Geometry check sheet. Reference: the model listing, model coordinates, mm. Give positions to 0.01 mm unless a question says otherwise; leave off trailing zeros. Order: outer loops, then holes, each group sorted by start corner. A loop starts at its lowest first (then second) coordinate and runs counter-clockwise, first axis right, second up. Notation, with made-up numbers: M -25.75,23 L 1.25,23 A22 cw 1.25,33 Z; hole C 57,6.25 d7. An arc over 180 degrees is marked long. One line per question, with ' | ' between items. Start each with the question number.
from build123d import *

# Parameters (mm, degrees)
CROQUIS1_R                   = 2.5
SALIENTE_EXTRUIR1_DEPTH      = 4
CROQUIS2_W                   = 50
CROQUIS2_H                   = 4
SALIENTE_EXTRUIR2_DEPTH      = 20
SALIENTE_EXTRUIR3_DEPTH      = 3
SALIENTE_EXTRUIR3_DEPTH_BACK = 53
CROQUIS4_W                   = 23
CROQUIS4_H                   = 20
CORTAR_EXTRUIR1_DEPTH        = 20
CROQUIS5_R                   = 3
CORTAR_EXTRUIR2_DEPTH        = 17
CROQUIS6_R                   = 2.5
CORTAR_EXTRUIR3_DEPTH        = 20


with BuildPart() as part:
    # Croquis1 → Saliente-Extruir1 (new body)
    with BuildSketch(Plane(origin=(0, 0, 0), x_dir=(1, 0, 0), z_dir=(0, 1, 0))):
        Polygon((0, 0), (0, 20), (50, 20), (50, 0), (50, -4), (0, -4), align=None)
        with Locations(Location((10, 10, 0), (0, 0, 270))):
            Circle(CROQUIS1_R, mode=Mode.SUBTRACT)
        with Locations(Location((40, 10, 0), (0, 0, 270))):
            Circle(CROQUIS1_R, mode=Mode.SUBTRACT)
    extrude(amount=SALIENTE_EXTRUIR1_DEPTH)

    # Croquis2 → Saliente-Extruir2 (add)
    with BuildSketch(Plane(origin=(0, 4, 0), x_dir=(1, 0, 0), z_dir=(0, 1, 0))):
        with Locations((25, -2)):
            Rectangle(CROQUIS2_W, CROQUIS2_H)
    extrude(amount=SALIENTE_EXTRUIR2_DEPTH)

    # Croquis3 → Saliente-Extruir3 (add, two sides: drawn at the far end of the back side and taken through both)
    with BuildSketch(Plane.ZY.offset(-SALIENTE_EXTRUIR3_DEPTH_BACK)):
        Polygon((-20, 4), (-20, 0), (4, 0), (4, 24), (0, 24), align=None)
    extrude(amount=SALIENTE_EXTRUIR3_DEPTH + SALIENTE_EXTRUIR3_DEPTH_BACK)

    # Croquis4 → Cortar-Extruir1 (cut)
    with BuildSketch(Plane(origin=(0, 0, -20), x_dir=(-1, 0, 0), z_dir=(0, 0, -1))):
        with Locations((-39, 14)):
            Rectangle(CROQUIS4_W, CROQUIS4_H)
        with Locations((-11, 14)):
            Rectangle(CROQUIS4_W, CROQUIS4_H)
    extrude(amount=-CORTAR_EXTRUIR1_DEPTH, mode=Mode.SUBTRACT)

    # Croquis5 → Cortar-Extruir2 (cut)
    with BuildSketch(Plane(origin=(0, 0, 0), x_dir=(-1, 0, 0), z_dir=(0, 0, -1))):
        with Locations((-40, 14)):
            Circle(CROQUIS5_R)
        with Locations((-10, 14)):
            Circle(CROQUIS5_R)
    extrude(amount=-CORTAR_EXTRUIR2_DEPTH, mode=Mode.SUBTRACT)

    # Croquis6 → Cortar-Extruir3 (cut)
    with BuildSketch(Plane(origin=(0, 4, 0), x_dir=(1, 0, 0), z_dir=(0, 1, 0))):
        with Locations(Location((10, 10, 0), (0, 0, 180))):
            Circle(CROQUIS6_R)
        with Locations(Location((40, 10, 0), (0, 0, 180))):
            Circle(CROQUIS6_R)
    extrude(amount=-CORTAR_EXTRUIR3_DEPTH, mode=Mode.SUBTRACT)

    # Croquis7 → Cortar-Revolución1 (revolve, cut)
    with BuildSketch(Plane.XY.offset(-10), mode=Mode.PRIVATE) as cortar_revoluci_n1_sk:
        Polygon((40, 0.7), (37.5, 0.7), (34.2, 4), (40, 4), align=None)
    revolve(cortar_revoluci_n1_sk.sketch.rotate(Axis((40, 0.7, -10), (0, 1, 0)), 270), axis=Axis((40, 0.7, -10), (0, 1, 0)), mode=Mode.SUBTRACT)

    # Croquis8 → Cortar-Revolución2 (revolve, cut)
    with BuildSketch(Plane.XY.offset(-10), mode=Mode.PRIVATE) as cortar_revoluci_n2_sk:
        Polygon((10, 4), (10, 0.7), (12.5, 0.7), (15.8, 4), align=None)
    revolve(cortar_revoluci_n2_sk.sketch.rotate(Axis((10, 4, -10), (0, -1, 0)), 90), axis=Axis((10, 4, -10), (0, -1, 0)), mode=Mode.SUBTRACT)

    # Croquis9 → Cortar-Revolución3 (revolve, cut)
    with BuildSketch(Plane(origin=(0, 14, 0), x_dir=(1, 0, 0), z_dir=(0, 1, 0)), mode=Mode.PRIVATE) as cortar_revoluci_n3_sk:
        Polygon((40, 0), (40, -3.3), (43, -3.3), (46.3, 0), align=None)
    revolve(cortar_revoluci_n3_sk.sketch.rotate(Axis((40, 14, 0), (0, 0, 1)), 180), axis=Axis((40, 14, 0), (0, 0, 1)), mode=Mode.SUBTRACT)

    # Croquis10 → Cortar-Revolución4 (revolve, cut)
    with BuildSketch(Plane(origin=(0, 14, 0), x_dir=(1, 0, 0), z_dir=(0, 1, 0)), mode=Mode.PRIVATE) as cortar_revoluci_n4_sk:
        Polygon((10, 0), (10, -3.3), (13, -3.3), (16.3, 0), align=None)
    revolve(cortar_revoluci_n4_sk.sketch.rotate(Axis((10, 14, 0), (0, 0, 1)), 180), axis=Axis((10, 14, 0), (0, 0, 1)), mode=Mode.SUBTRACT)


solid = part.part
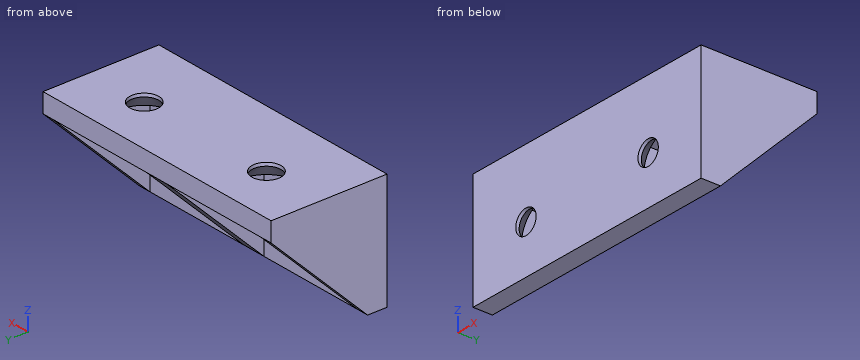
Item 1: Cross-section at C-C, the plane y = 14. Record the cut outline in (x, z).
Item 2: Cross-section at B-B, the plane z = -10. Record the cut outline in (x, y), plus the area to 3 significant figures.
Item 3: Depth check by flat-ended pin: pin 1 (3 mm diameter, centred on x = 47, z = -12, fed in from +Y); pin 2 (6 mm diameter, centred on x = 38.5, y = 18, fed in from -Z); pin 3 (6 mm diameter, centred on x = 11.5, z = -8, fed in from +Y); pin 4 (6 mm diameter, centred on y = 14, z = -17, fed in from -X). Enter the tip coordinate at first touch or a pass-through.
Item 4: Cross-section at D-D, the plane z = -3. Record the cut outline in (x, y), plus the area to 3 significant figures.
Item 5: Material ranges on line 1 along X through (y, z) = (0.2, -10); line 2 along X through (y, z) = (17.25, -6); line 3 along Y through (x, z) = (40, 3.8), recorded low to high.
Item 6: Cross-section at A-A, the plane x = 40. Record the cut outline in (y, z).
Outcome:
1) outline: M -3,-10 L -0.5,-10 L -0.5,0 L 3.7,0 L 7,3.3 L 7,4 L -3,4 Z; M 13,3.3 L 16.3,0 L 22.5,0 L 22.5,-10 L 27.5,-10 L 27.5,0 L 33.7,0 L 37,3.3 L 37,4 L 13,4 Z; M 43,3.3 L 46.3,0 L 50.5,0 L 50.5,-10 L 53,-10 L 53,4 L 43,4 Z
2) outline: M -3,0 L 7.5,0 L 7.5,0.7 L 4.2,4 L -0.5,4 L -0.5,14 L -3,14 Z; M 12.5,0 L 37.5,0 L 37.5,0.7 L 34.2,4 L 27.5,4 L 27.5,14 L 22.5,14 L 22.5,4 L 15.8,4 L 12.5,0.7 Z; M 42.5,0 L 53,0 L 53,14 L 50.5,14 L 50.5,4 L 45.8,4 L 42.5,0.7 Z | area: 262 mm²
3) pin 1: stops at y = 4 | pin 2: stops at z = 0 | pin 3: stops at y = 3.7 | pin 4: passes through
4) outline: M -3,0 L 53,0 L 53,21 L 50.5,21 L 50.5,4 L 27.5,4 L 27.5,21 L 22.5,21 L 22.5,4 L -0.5,4 L -0.5,21 L -3,21 Z | area: 394 mm²
5) line 1: x = -3 to 7.5, 12.5 to 37.5, 42.5 to 53 | line 2: x = -3 to -0.5, 22.5 to 27.5, 50.5 to 53 | line 3: y = 0 to 11, 17 to 24
6) outline: M 0,-20 L 4,-20 L 4,-15.8 L 0.7,-12.5 L 0,-12.5 Z; M 0,-7.5 L 0.7,-7.5 L 4,-4.2 L 4,0 L 7.7,0 L 11,3.3 L 11,4 L 0,4 Z; M 17,3.3 L 20.3,0 L 24,0 L 24,4 L 17,4 Z
